```python
from build123d import *

# Parameters (mm, degrees)
BOSS_EXTRUDE1_DEPTH     = 35
SKETCH2_R               = 4
CUT_EXTRUDE1_DEPTH      = 101
SKETCH3_R               = 7.5
SKETCH3_R_2             = 5
CUT_EXTRUDE2_DEPTH      = 1
CUT_EXTRUDE2_DEPTH_BACK = 71
CHAMFER1_SIZE           = 12
CHAMFER1_SIZE2          = 6.92820323
CHAMFER2_SIZE           = 12
CHAMFER2_SIZE2          = 6.92820323
SKETCH4_R               = 10
CUT_EXTRUDE3_DEPTH      = 12
CUT_EXTRUDE4_START      = -18.803848
SKETCH5_R               = 1.5
CUT_EXTRUDE4_DEPTH      = 18.803848
BOSS_EXTRUDE2_DEPTH     = 12
SKETCH7_R               = 2.75
CUT_EXTRUDE5_DEPTH      = 41
SKETCH8_R               = 10
SKETCH8_R_2             = 1.5
BOSS_EXTRUDE3_DEPTH     = 12
SKETCH9_R               = 8.5
CUT_EXTRUDE6_DEPTH      = 6
SKETCH10_R              = 11
CUT_EXTRUDE7_DEPTH      = 4
SKETCH11_R              = 5
SKETCH11_R_2            = 1.1
CUT_EXTRUDE8_DEPTH      = 20


with BuildPart() as part:
    # Sketch1 → Boss-Extrude1 (new body, symmetric)
    with BuildSketch(Plane(origin=(0, 0, 0), x_dir=(0, 0, -1), z_dir=(1, 0, 0))):
        Polygon((30, 50), (30, -50), (-41, -50), (-41, -38), (0, -38), (0, 38), (-41, 38), (-41, 50), align=None)
    extrude(amount=BOSS_EXTRUDE1_DEPTH, both=True)

    # Sketch2 → Cut-Extrude1 (cut, through all)
    with BuildSketch(Plane(origin=(0, 50, 0), x_dir=(1, 0, 0), z_dir=(0, 1, 0))):
        with Locations((-22.5, -20)):
            Circle(SKETCH2_R)
        with Locations((22.5, -20)):
            Circle(SKETCH2_R)
        with Locations((0, -20)):
            Circle(SKETCH2_R)
    extrude(amount=-CUT_EXTRUDE1_DEPTH, mode=Mode.SUBTRACT)

    # Sketch3 → Cut-Extrude2 (cut, two sides)
    with BuildSketch(Plane(origin=(35, 0, 0), x_dir=(0, 0, -1), z_dir=(1, 0, 0))) as cut_extrude2_sk:
        with Locations((15, -37.25)):
            Circle(SKETCH3_R)
        with Locations((15, 37.25)):
            Circle(SKETCH3_R)
        with Locations((14.2, 0)):
            Circle(SKETCH3_R_2)
    extrude(amount=CUT_EXTRUDE2_DEPTH, mode=Mode.SUBTRACT)
    extrude(cut_extrude2_sk.sketch, amount=-CUT_EXTRUDE2_DEPTH_BACK, mode=Mode.SUBTRACT)

    # Chamfer1
    chamfer1_edges = [part.edges().sort_by_distance(p)[0] for p in [
        (0, -38, 0),
    ]]
    chamfer1_side = [part.faces().sort_by_distance(p)[0] for p in [
        (0, 0, 0),
    ]]
    chamfer(chamfer1_edges, length=CHAMFER1_SIZE, length2=CHAMFER1_SIZE2, reference=chamfer1_side[0])

    # Chamfer2
    chamfer2_edges = [part.edges().sort_by_distance(p)[0] for p in [
        (0, 38, 0),
    ]]
    chamfer2_side = [part.faces().sort_by_distance(p)[0] for p in [
        (0, 6, 0),
    ]]
    chamfer(chamfer2_edges, length=CHAMFER2_SIZE, length2=CHAMFER2_SIZE2, reference=chamfer2_side[0])

    # Sketch4 → Cut-Extrude3 (cut)
    with BuildSketch(Plane(origin=(0, 50, 0), x_dir=(1, 0, 0), z_dir=(0, 1, 0))):
        with Locations((0, -20)):
            Circle(SKETCH4_R)
    extrude(amount=-CUT_EXTRUDE3_DEPTH, mode=Mode.SUBTRACT)

    # Sketch5 → Cut-Extrude4 (cut)
    with BuildSketch(Plane(origin=(0, 50, 0), x_dir=(1, 0, 0), z_dir=(0, 1, 0)).offset(CUT_EXTRUDE4_START)):
        with Locations((15.5, -4.5)):
            Circle(SKETCH5_R)
        with Locations((-15.5, -4.5)):
            Circle(SKETCH5_R)
        with Locations((15.5, -35.5)):
            Circle(SKETCH5_R)
        with Locations((-15.5, -35.5)):
            Circle(SKETCH5_R)
    extrude(amount=CUT_EXTRUDE4_DEPTH, mode=Mode.SUBTRACT)

    # Sketch6 → Boss-Extrude2 (add, symmetric)
    with BuildSketch(Plane(origin=(0, 50, 0), x_dir=(1, 0, 0), z_dir=(0, 1, 0))):
        with BuildLine():
            Line((-21.309475019, -41), (-9.690524981, -41))
            ThreePointArc((-9.690524981, -41), (-15.5, -43.5), (-21.309475019, -41))
        make_face()
        with BuildLine():
            Line((21.309475019, -41), (9.690524981, -41))
            ThreePointArc((9.690524981, -41), (15.5, -43.5), (21.309475019, -41))
        make_face()
    extrude(amount=BOSS_EXTRUDE2_DEPTH, both=True)

    # Sketch7 → Cut-Extrude5 (cut)
    with BuildSketch(Plane(origin=(0, 0, 0), x_dir=(1, 0, 0), z_dir=(0, 1, 0))):
        with Locations((15.5, -4.5)):
            Circle(SKETCH7_R)
        with Locations((-15.5, -4.5)):
            Circle(SKETCH7_R)
        with Locations((15.5, -35.5)):
            Circle(SKETCH7_R)
        with Locations((-15.5, -35.5)):
            Circle(SKETCH7_R)
    extrude(amount=CUT_EXTRUDE5_DEPTH, mode=Mode.SUBTRACT)

    # Sketch8 → Boss-Extrude3 (add)
    with BuildSketch(Plane(origin=(0, 50, 0), x_dir=(1, 0, 0), z_dir=(0, 1, 0))):
        Polygon((17.464466094, 1), (-17.464466094, 1), (-21, 1), (-21, -2.535533906), (-21, -37.464466094), (-21, -41), (-17.464466094, -41), (17.464466094, -41), (21, -41), (21, -37.464466094), (21, -2.535533906), (21, 1), align=None)
        with Locations((0, -20)):
            Circle(SKETCH8_R, mode=Mode.SUBTRACT)
        with Locations((-15.5, -35.5)):
            Circle(SKETCH8_R_2, mode=Mode.SUBTRACT)
        with Locations((15.5, -35.5)):
            Circle(SKETCH8_R_2, mode=Mode.SUBTRACT)
        with Locations((-15.5, -4.5)):
            Circle(SKETCH8_R_2, mode=Mode.SUBTRACT)
        with Locations((15.5, -4.5)):
            Circle(SKETCH8_R_2, mode=Mode.SUBTRACT)
    extrude(amount=BOSS_EXTRUDE3_DEPTH)

    # Sketch9 → Cut-Extrude6 (cut)
    with BuildSketch(Plane(origin=(0, -38, 0), x_dir=(1, 0, 0), z_dir=(0, 1, 0))):
        with Locations((0, -20)):
            Circle(SKETCH9_R)
    extrude(amount=-CUT_EXTRUDE6_DEPTH, mode=Mode.SUBTRACT)

    # Sketch10 → Cut-Extrude7 (cut)
    with BuildSketch(Plane.ZY.offset(35)):
        with Locations((-14.2, 0)):
            Circle(SKETCH10_R)
    extrude(amount=-CUT_EXTRUDE7_DEPTH, mode=Mode.SUBTRACT)

    # Sketch11 → Cut-Extrude8 (cut)
    with BuildSketch(Plane.ZY.offset(31)):
        with Locations((-14.2, 0)):
            Circle(SKETCH11_R)
        with Locations((-14.2, 8)):
            Circle(SKETCH11_R_2)
        with Locations((-6.2, 0)):
            Circle(SKETCH11_R_2)
        with Locations((-14.2, -8)):
            Circle(SKETCH11_R_2)
        with Locations((-22.2, 0)):
            Circle(SKETCH11_R_2)
    extrude(amount=-CUT_EXTRUDE8_DEPTH, mode=Mode.SUBTRACT)


solid = part.part
```
Read the model definition and answer for the solid it produces. Units are mm, in the model's axes. A direction names the side the tool comes from. Give positions to 0.01 mm unless a question says otherwise; leave off trailing zeros. Write each loop counter-clockwise with the first axis right and the second up, starting at its lowest first coordinate (ties: lowest second). Pieces come first, ordered by that corner, then holes. Notation, with made-up numbers: (-35.75, -38) - (-23.75, -38) arc R9 ccw to (-23.75, -21) - close; hole circle Ø6 at (-25.75, -2). An arc over 180 degrees is marked (long way). Write item = value, one per line. Start each with the question number.
Item 1: Find section A-A (x = -15.5). State how many separate pieces and enclosed holes the cut face has, then the cut area to 3 significant figures.
Item 2: Find section C-C (z = 35.5). Give the vertices of the cut face in (x, y), then the cut area to 4 significant figures.
Item 3: Find section D-D (y = -42.5). Give the vertices of the cut face in (x, z).
Item 4: Each of these flat-tipped pins is pushed along its axis until it touches: P1, Ø3.5, axis at x = -25.5, y = 46, coming from the +Z side; P2, Ø3.5, axis at y = 53, z = 11.5, coming from the -X side; P3, Ø10.5, axis at x = 22.5, z = 20, coming from the -Y side; P4, Ø1.8, axis at y = 0.5, z = -6, coming from the -X side. Where does it stop, or does it pass through?
Item 5: Find section B-B (y = 47). Give the vertices of the cut face in (x, z).
Item 6: The mould has two halves that part along Z. Classify faces 4 (the flat face through (0.49, 32.08, 3.51)), 5 (the flat face through (-14, 41, 37)), 6 (the flat face through (21, 56, 20)): +Z half, -Z half, draft (parallel to the pull), parting line (faces both ways), or undercut.
Item 7: Find the intervals of material crossed by probe 1 along X at (y, z) = (52, 4.5); probe 2 along X at (y, z) = (-41, 20); probe 3 along X at (y, z) = (40, 20), in increasing order. Write a range as [from, to].
Item 8: A tool of negligible diameter and unlimited length cuts with its end or side. For faces 1 (the cylindrical face through (-16.7, 51.4, 36.4)), 2 (the flat face through (-31, -5, -12)), 3 (the flat face through (-28, 44, 41)), from which of +Z, -Z, +X, -X, +Y, -Y can it reach the whole face along a straight path? Write none if from no direction.
Response:
q1.separate_pieces = 3
q1.enclosed_holes = 7
q1.area = 4,000 mm²
q2.outline = (-35, -50) - (35, -50) - (35, -38) - (-35, -38) - close; (-35, 38) - (-18.25, 38) - (-18.25, 41) - (-17, 41) - (-17, 62) - (-21, 62) - (-21, 50) - (-35, 50) - close; (-14, 41) - (-12.75, 41) - (-12.75, 38) - (12.75, 38) - (12.75, 41) - (14, 41) - (14, 62) - (-14, 62) - close; (17, 41) - (18.25, 41) - (18.25, 38) - (35, 38) - (35, 50) - (21, 50) - (21, 62) - (17, 62) - close
q2.area = 2,025 mm²
q3.outline = (-35, -30) - (35, -30) - (35, -20.36) - (-35, -20.36) - close; (-35, -9.64) - (35, -9.64) - (35, 41) - (-35, 41) - close; hole circle Ø8 at (-22.5, 20); hole circle Ø17 at (0, 20); hole circle Ø8 at (22.5, 20)
q4.P1 = 41
q4.P2 = -21
q4.P3 = -50
q4.P4 = -31
q5.outline = (-35, -30) - (35, -30) - (35, 41) - (21.31, 41) arc R8 ccw to (9.69, 41) - (-9.69, 41) arc R8 ccw to (-21.31, 41) - (-35, 41) - close; hole circle Ø8 at (-22.5, 20); hole circle Ø3 at (-15.5, 4.5); hole circle Ø3 at (-15.5, 35.5); hole circle Ø20 at (0, 20); hole circle Ø3 at (15.5, 4.5); hole circle Ø3 at (15.5, 35.5); hole circle Ø8 at (22.5, 20)
q6.face_4 = +Z half
q6.face_5 = undercut
q6.face_6 = draft
q7.probe_1 = [-21, -17], [-14, 14], [17, 21]
q7.probe_2 = [-35, -26.5], [-18.5, -8.5], [8.5, 18.5], [26.5, 35]
q7.probe_3 = [-35, -26.5], [-18.5, -10], [10, 18.5], [26.5, 35]
q8.face_1 = +Y
q8.face_2 = -X
q8.face_3 = +Z, -X, +Y, -Y
